For this review, take the finished solid that the model builds, in its own axes (mm). A direction names the side the tool comes from. Coordinates: 2 decimals unless noted, no trailing zeros. Order: outer loops, then holes, each group sorted by start corner. A loop starts at its lowest first (then second) coordinate and runs counter-clockwise, first axis right, second up. Notation, with made-up numbers: (-7.5, 5) -> (20.5, 5) arc R17 ccw to (20.5, 9) -> close; hole circle Ø9 at (2.25, 13.25). An arc over 180 degrees is marked (long way). Answer as a JSON object with one key per item and string values. Group by question number.
1) Draft analysis for pull direction X (two halves, no side actions). For faces 1 (the flat face through (9, 21.5, 3)), 2 (the flat face through (-72.5, 15, 1)), 3 (the flat face through (-1, 15, 72.5)), state which applies: +X half, -X half, draft (parallel to the pull), parting line (faces both ways), or undercut.
2) Wall thickness on L1, parallel to X at y = 21, z = -58; L2, parallel to X at y = 21.75, z = 39; L3, parallel to Z at x = 62, y = 18.25: over which ranges is each line inside the solid? List them lowest first.
3) Add section B-B, the plane z = 0. Write out the cut boundary in (x, y), then the cut area to 3 significant figures.
4) Add section D-D, the plane x = -39.5. Write out the cut boundary in (y, z), then the cut area to 3 significant figures.
5) Add section A-A, the plane y = 10. Write out the cut boundary in (x, z).
6) Machinability: for faces 4 (the flat face through (-1, 15, -72.5)), 5 (the flat face through (5.413, 17, 0)), which of the approach directions +Z, -Z, +X, -X, +Y, -Y give a long, thin tool a straight path to every point of the face, cutting with its end or side? Answer none if there is none.
7) Add section C-C, the plane y = 18. Write out the cut boundary in (x, z) (3 decimals).
8) For pin 1 (7 mm diameter, centred on x = 6, z = -2, fed in from +Y); pin 2 (6 mm diameter, centred on x = 17.5, z = -4.5, fed in from +Y); pin 3 (8 mm diameter, centred on x = 0, z = 0, fed in from +Y), all flat-tipped, find the tip position at first contact; note any pin that passes through.
from build123d import *

# Parameters (mm, degrees)
SKETCH1_W           = 145
SKETCH1_H           = 145
BOSS_EXTRUDE1_DEPTH = 30
SKETCH2_W           = 87
SKETCH2_H           = 87
CUT_EXTRUDE1_DEPTH  = 22.5
SKETCH3_R           = 12
BOSS_EXTRUDE2_DEPTH = 14
CUT_EXTRUDE2_DEPTH  = 7
SKETCH5_R           = 5.5
CUT_EXTRUDE3_DEPTH  = 15
CUT_EXTRUDE4_REACH  = 105.695
SKETCH6_R           = 3.05
SKETCH7_R           = 9.15
CUT_EXTRUDE5_DEPTH  = 1.5


with BuildPart() as part:
    # Sketch1 → Boss-Extrude1 (new body)
    with BuildSketch(Plane(origin=(0, 0, 0), x_dir=(1, 0, 0), z_dir=(0, 1, 0))):
        Rectangle(SKETCH1_W, SKETCH1_H)
    extrude(amount=BOSS_EXTRUDE1_DEPTH)

    # Sketch2 → Cut-Extrude1 (cut)
    with BuildSketch(Plane(origin=(0, 30, 0), x_dir=(1, 0, 0), z_dir=(0, 1, 0))):
        Rectangle(SKETCH2_W, SKETCH2_H)
    extrude(amount=-CUT_EXTRUDE1_DEPTH, mode=Mode.SUBTRACT)

    # Sketch3 → Boss-Extrude2 (add)
    with BuildSketch(Plane(origin=(0, 7.5, 0), x_dir=(1, 0, 0), z_dir=(0, 1, 0))):
        with Locations(Location((0, 0, 0), (0, 0, 90))):
            Circle(SKETCH3_R)
    extrude(amount=BOSS_EXTRUDE2_DEPTH)

    # Sketch4 → Cut-Extrude2 (cut)
    with BuildSketch(Plane(origin=(0, 21.5, 0), x_dir=(1, 0, 0), z_dir=(0, 1, 0))):
        Polygon((0, 6.25), (-5.412658774, 3.125), (-5.412658774, -3.125), (0, -6.25), (5.412658774, -3.125), (5.412658774, 3.125), align=None)
    extrude(amount=-CUT_EXTRUDE2_DEPTH, mode=Mode.SUBTRACT)

    # Sketch5 → Cut-Extrude3 (cut)
    with BuildSketch(Plane(origin=(0, 30, 0), x_dir=(1, 0, 0), z_dir=(0, 1, 0))):
        with Locations(Location((-58, 58, 0), (0, 0, 270))):
            Circle(SKETCH5_R)
        with Locations(Location((58, 58, 0), (0, 0, 90))):
            Circle(SKETCH5_R)
        with Locations(Location((58, -58, 0), (0, 0, 270))):
            Circle(SKETCH5_R)
        with Locations(Location((-58, -58, 0), (0, 0, 90))):
            Circle(SKETCH5_R)
    extrude(amount=-CUT_EXTRUDE3_DEPTH, mode=Mode.SUBTRACT)

    # Sketch6 → Cut-Extrude4 (cut, up to next)
    with BuildSketch(Plane(origin=(0, 14.5, 0), x_dir=(1, 0, 0), z_dir=(0, 1, 0)), mode=Mode.PRIVATE) as cut_extrude4_sk1:
        with Locations(Location((0, 0, 0), (0, 0, 270))):
            Circle(SKETCH6_R)
    cut_extrude4_tool1 = extrude(cut_extrude4_sk1.sketch, amount=-CUT_EXTRUDE4_REACH, mode=Mode.PRIVATE) & part.part
    add(cut_extrude4_tool1.solids().sort_by_distance((0, 14.5, 0))[0], mode=Mode.SUBTRACT)

    # Sketch7 → Cut-Extrude5 (cut)
    with BuildSketch(Plane(origin=(0, 21.5, 0), x_dir=(1, 0, 0), z_dir=(0, 1, 0))):
        with Locations(Location((0, 0, 0), (0, 0, 270))):
            Circle(SKETCH7_R)
    extrude(amount=-CUT_EXTRUDE5_DEPTH, mode=Mode.SUBTRACT)


solid = part.part
Output values:
{
 "1": {"face 1": "undercut", "face 2": "-X half", "face 3": "draft"},
 "2": {"L1": "x = -72.5 to -63.5, -52.5 to 52.5, 63.5 to 72.5", "L2": "x = -72.5 to -43.5, 43.5 to 72.5", "L3": "z = -72.5 to -61.77, -54.23 to 54.23, 61.77 to 72.5"},
 "3": {"outline": "(-72.5, 0) -> (-3.05, 0) -> (-3.05, 14.5) -> (-5.41, 14.5) -> (-5.41, 20) -> (-9.15, 20) -> (-9.15, 21.5) -> (-12, 21.5) -> (-12, 7.5) -> (-43.5, 7.5) -> (-43.5, 30) -> (-72.5, 30) -> close; (3.05, 0) -> (72.5, 0) -> (72.5, 30) -> (43.5, 30) -> (43.5, 7.5) -> (12, 7.5) -> (12, 21.5) -> (9.15, 21.5) -> (9.15, 20) -> (5.41, 20) -> (5.41, 14.5) -> (3.05, 14.5) -> close", "area": "2,550 mm²"},
 "4": {"outline": "(0, -72.5) -> (30, -72.5) -> (30, -43.5) -> (7.5, -43.5) -> (7.5, 43.5) -> (30, 43.5) -> (30, 72.5) -> (0, 72.5) -> close", "area": "2,390 mm²"},
 "5": {"outline": "(-72.5, -72.5) -> (72.5, -72.5) -> (72.5, 72.5) -> (-72.5, 72.5) -> close; circle Ø24 at (0, 0); hole (-43.5, -43.5) -> (43.5, -43.5) -> (43.5, 43.5) -> (-43.5, 43.5) -> close; hole circle Ø6.1 at (0, 0)"},
 "6": {"face 4": "-Z, +X, -X, +Y, -Y", "face 5": "+Y"},
 "7": {"outline": "(-72.5, -72.5) -> (72.5, -72.5) -> (72.5, 72.5) -> (-72.5, 72.5) -> close; circle Ø24 at (0, 0); hole circle Ø11 at (-58, -58); hole circle Ø11 at (-58, 58); hole (-43.5, -43.5) -> (43.5, -43.5) -> (43.5, 43.5) -> (-43.5, 43.5) -> close; hole (-5.413, -3.125) -> (0, -6.25) -> (5.413, -3.125) -> (5.413, 3.125) -> (0, 6.25) -> (-5.413, 3.125) -> close; hole circle Ø11 at (58, -58); hole circle Ø11 at (58, 58)"},
 "8": {"pin 1": "stops at y = 21.5", "pin 2": "stops at y = 7.5", "pin 3": "stops at y = 14.5"}
}
